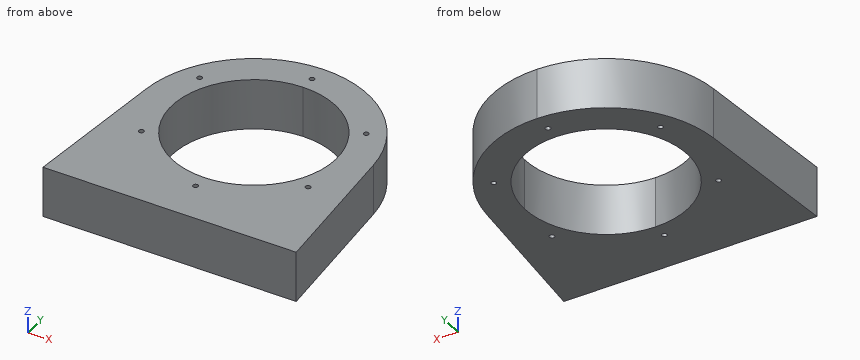
```python
from build123d import *

# Parameters (mm, degrees)
EXTRUDE_1_DEPTH     = 30
CUT_EXTRUDE_1_REACH = 216.243
SKETCH_2_R          = 1.5


with BuildPart() as part:
    # 草图1 → 凸台-拉伸1 (new body)
    with BuildSketch(Plane.XY):
        with BuildLine():
            Line((7.726793577, 88.353296402), (0, 0))
            Line((0, 0), (75, 0))
            Line((75, 0), (75, 34.220027747))
            ThreePointArc((75, 34.220027747), (26.75, 82.470027747), (75, 130.720027747))
            Line((75, 130.720027747), (75, 150))
            ThreePointArc((75, 150), (29.376540117, 132.257546873), (7.726793577, 88.353296402))
        make_face()
        with BuildLine():
            Line((75, 34.220027747), (75, 0))
            Line((75, 0), (150, 0))
            Line((150, 0), (142.273206423, 88.353296402))
            ThreePointArc((142.273206423, 88.353296402), (120.623459883, 132.257546873), (75, 150))
            Line((75, 150), (75, 130.720027747))
            ThreePointArc((75, 130.720027747), (109.117902192, 116.587929939), (123.25, 82.470027747))
            ThreePointArc((123.25, 82.470027747), (109.117902192, 48.352125555), (75, 34.220027747))
        make_face()
    extrude(amount=EXTRUDE_1_DEPTH)

    # 草图2 → 切除-拉伸1 (cut, up to next)
    with BuildSketch(Plane.XY.offset(30), mode=Mode.PRIVATE) as cut_extrude_1_sk1:
        with Locations((75, 139.470027747)):
            Circle(SKETCH_2_R)
    cut_extrude_1_tool1 = extrude(cut_extrude_1_sk1.sketch, amount=-CUT_EXTRUDE_1_REACH, mode=Mode.PRIVATE) & part.part
    # 草图2 → 切除-拉伸1 (cut, up to next)
    with BuildSketch(Plane.XY.offset(30), mode=Mode.PRIVATE) as cut_extrude_1_sk2:
        with Locations((124.363448016, 110.970027747)):
            Circle(SKETCH_2_R)
    cut_extrude_1_tool2 = extrude(cut_extrude_1_sk2.sketch, amount=-CUT_EXTRUDE_1_REACH, mode=Mode.PRIVATE) & part.part
    # 草图2 → 切除-拉伸1 (cut, up to next)
    with BuildSketch(Plane.XY.offset(30), mode=Mode.PRIVATE) as cut_extrude_1_sk3:
        with Locations((124.363448016, 53.970027747)):
            Circle(SKETCH_2_R)
    cut_extrude_1_tool3 = extrude(cut_extrude_1_sk3.sketch, amount=-CUT_EXTRUDE_1_REACH, mode=Mode.PRIVATE) & part.part
    # 草图2 → 切除-拉伸1 (cut, up to next)
    with BuildSketch(Plane.XY.offset(30), mode=Mode.PRIVATE) as cut_extrude_1_sk4:
        with Locations((75, 25.470027747)):
            Circle(SKETCH_2_R)
    cut_extrude_1_tool4 = extrude(cut_extrude_1_sk4.sketch, amount=-CUT_EXTRUDE_1_REACH, mode=Mode.PRIVATE) & part.part
    # 草图2 → 切除-拉伸1 (cut, up to next)
    with BuildSketch(Plane.XY.offset(30), mode=Mode.PRIVATE) as cut_extrude_1_sk5:
        with Locations((25.636551984, 53.970027747)):
            Circle(SKETCH_2_R)
    cut_extrude_1_tool5 = extrude(cut_extrude_1_sk5.sketch, amount=-CUT_EXTRUDE_1_REACH, mode=Mode.PRIVATE) & part.part
    # 草图2 → 切除-拉伸1 (cut, up to next)
    with BuildSketch(Plane.XY.offset(30), mode=Mode.PRIVATE) as cut_extrude_1_sk6:
        with Locations((25.636551984, 110.970027747)):
            Circle(SKETCH_2_R)
    cut_extrude_1_tool6 = extrude(cut_extrude_1_sk6.sketch, amount=-CUT_EXTRUDE_1_REACH, mode=Mode.PRIVATE) & part.part
    add(cut_extrude_1_tool1.solids().sort_by_distance((75, 139.470028, 30))[0], mode=Mode.SUBTRACT)
    add(cut_extrude_1_tool2.solids().sort_by_distance((124.363448, 110.970028, 30))[0], mode=Mode.SUBTRACT)
    add(cut_extrude_1_tool3.solids().sort_by_distance((124.363448, 53.970028, 30))[0], mode=Mode.SUBTRACT)
    add(cut_extrude_1_tool4.solids().sort_by_distance((75, 25.470028, 30))[0], mode=Mode.SUBTRACT)
    add(cut_extrude_1_tool5.solids().sort_by_distance((25.636552, 53.970028, 30))[0], mode=Mode.SUBTRACT)
    add(cut_extrude_1_tool6.solids().sort_by_distance((25.636552, 110.970028, 30))[0], mode=Mode.SUBTRACT)


solid = part.part
```
CAD build for the part. Positions are in the model's coordinates, mm. Round coordinates to 2 decimals unless told otherwise and drop trailing zeros. Write each loop counter-clockwise with the first axis right and the second up, starting at its lowest first coordinate (ties: lowest second). Pieces come first, ordered by that corner, then holes. Notation, with made-up numbers: M -9,-9.75 L 40,-9.75 A12 ccw 40,-4.75 Z; hole C 13.25,27.25 d9. An arc over 180 degrees is marked long. One line per question, with ' | ' between items.
1. Cut at D-D on x = 130. Write the cut outline in (y, z), and give its area (3 significant figures).
Working result:
outline: M 0,0 L 121.65,0 L 121.65,30 L 0,30 Z | area: 3,650 mm2
2. Probe L1, parallel to Y at x = 75, z = 24; L2, parallel to X at y = 55, z = 16; L3, parallel to X at y = 140, z = 10.75. List the from-to ranges inside material, lowest first. Write a range as from..to.
Working result:
L1: 0..23.97, 26.97..34.22, 130.72..137.97, 140.97..150 | L2: 4.81..24.55, 26.73..35.33, 114.67..123.27, 125.45..145.19 | L3: 39.64..73.6, 76.4..110.36
3. Cut at A-A on y = 122.5. Write the cut outline in (x, z).
Working result:
outline: M 20.61,0 L 48.06,0 L 48.06,30 L 20.61,30 Z; M 101.94,0 L 129.39,0 L 129.39,30 L 101.94,30 Z
4. Cut at B-B on x = 109. Write the cut outline in (y, z), and give its area (3 significant figures).
Working result:
outline: M 0,0 L 48.23,0 L 48.23,30 L 0,30 Z; M 116.71,0 L 140.82,0 L 140.82,30 L 116.71,30 Z | area: 2,170 mm2
5. Pin check, flat tips, straight feed: pin 1 Ø1.8 at (x, y) = (75, 139.47) entering from -Z; pin 2 Ø8 at (x, z) = (119.5, 9) entering from -Y; pin 3 Ø12 at (y, z) = (57.5, 18) entering from +X; pin 4 Ø6 at (y, z) = (133.5, 11) entering from -X. Stop position of each tip, or through.
Working result:
pin 1: through | pin 2: y = 0 | pin 3: x = 145.5 | pin 4: x = 27.53
6. Cut at C-C on z = 21.5. Write the cut outline in (x, y).
Working result:
outline: M 0,0 L 150,0 L 142.27,88.35 A67.53 ccw 7.73,88.35 Z; hole C 25.64,53.97 d3; hole C 25.64,110.97 d3; hole C 75,82.47 d96.5; hole C 75,25.47 d3; hole C 75,139.47 d3; hole C 124.36,53.97 d3; hole C 124.36,110.97 d3
